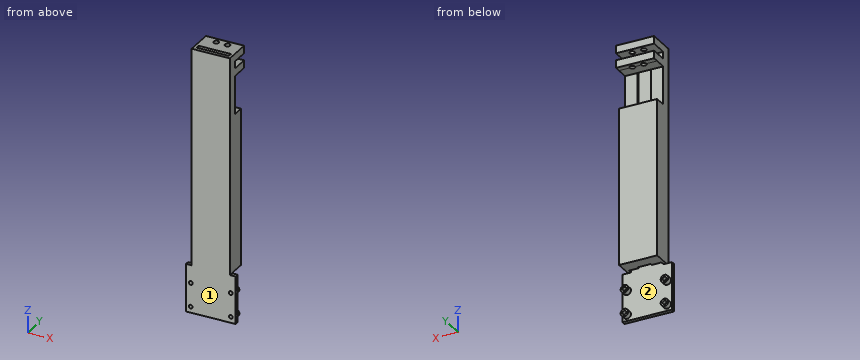
Autodesk Inventor part; units mm, degrees
ref_plane "YZ Plane" through (0, 0, 0) normal (1, 0, 0) x (0, 1, 0)
ref_plane "XZ Plane" through (0, 0, 0) normal (0, 1, 0) x (-1, 0, 0)
ref_plane "XY Plane" through (0, 0, 0) normal (0, 0, 1) x (1, 0, 0)
sketch "スケッチ1" plane through (0, 0, 0) normal (0, 1, 0) x (-1, 0, 0)
  line L0 (8.5, 24.0956) -> (-8.5, 24.0956)
  line L1 (-8.5, 24.0956) -> (-8.5, -85.9044)
  line L2 (-8.5, -85.9044) -> (8.5, -85.9044)
  line L3 (8.5, -85.9044) -> (8.5, 24.0956)
  line L4 (13, -85.9044) -> (-13, -85.9044)
  line L5 (-13, -85.9044) -> (-13, -110.9044)
  line L6 (-13, -110.9044) -> (13, -110.9044)
  line L7 (13, -110.9044) -> (13, -85.9044)
  circle A0 centre (10.5, -95.2644) radius 1
  circle A1 centre (10.5, -107.7644) radius 1
  line L8 (0, -85.9044) -> (0, -110.9044)
  line L9 (-8.5, -85.9044) -> (-8.5, 24.0956)
  circle A2 centre (-10.5, -95.2644) radius 1
  circle A3 centre (-10.5, -107.7644) radius 1
  line L10 (0, -85.9044) -> (0, 24.0956)
  line L11 (10, -85.9044) -> (10, 24.0956)
  line L12 (10, 24.0956) -> (8.5, 24.0956)
  line L13 (-8.5, -85.9044) -> (-8.5, 24.0956)
  line L14 (-10, -85.9044) -> (-10, 24.0956)
  line L15 (-10, 24.0956) -> (-8.5, 24.0956)
  line L16 (10, 24.0956) -> (-10, 24.0956)
  line L17 (8.5, 24.0956) -> (-8.5, 24.0956)
  line L18 (10, 24.0956) -> (-10, 24.0956)
  point P0 (0, 0)
  point P1 (-8.5, 24.0956)
  dimension "d0" = 17
  dimension "d1" = 110
  dimension "d2" = 26
  dimension "d3" = 25
  dimension "d4" = 4.5
  dimension "d5" = 2
  dimension "d6" = 9.36
  dimension "d7" = 2
  dimension "d8" = 12.5
  dimension "d9" = 2.5
  dimension "d10" = 2.5
  dimension "d11" = 13
  dimension "d12" = 1.5
extrude "押し出し1" add sketch "スケッチ1" along normal blind 2 contours L3 L2 L10 L0 | L10 L2 L1 L0 | L4 L7 L6 L8 L2 | L8 L6 L5 L4 L2
extrude "押し出し2" add sketch "スケッチ1" along normal blind 5 contours L12 L11 L4 L3 | L1 L4 L14 L15
sketch "スケッチ2" plane through (-8.5, 2, 24.0956) normal (1, 0, 0) x (0, 0, -1)
  line L0 (0, 0) -> (0, 3)
  line L1 (0, 3) -> (110, 3)
  line L2 (110, 3) -> (110, 2)
  line L3 (110, 2) -> (0, 2)
  line L4 (0, 2) -> (0, 3)
  point P0 (24.0956, -2)
  point P1 (0, 2)
  dimension "d27" = 110
  dimension "d28" = 1
sketch "スケッチ3" plane through (8.5, 2, -85.9044) normal (-1, 0, 0) x (0, 0, 1)
  line L0 (0, 3) -> (110, 3)
  line L1 (0, 3) -> (110, 3)
  line L2 (110, 3) -> (110, 2)
  line L3 (110, 2) -> (0, 2)
  line L4 (0, 2) -> (0, 3)
  point P0 (85.9044, -2)
  dimension "d29" = 110
  dimension "d30" = 1
sketch "スケッチ5" plane through (-10, 0, 24.0956) normal (0, 0, 1) x (1, 0, 0)
  line L0 (0, 0) -> (0, 2)
  line L1 (0, 0) -> (20, 0)
  line L2 (20, 0) -> (20, 14)
  line L3 (20, 14) -> (0, 14)
  line L4 (0, 14) -> (0, 0)
  line L5 (0, 2) -> (1.5, 2)
  line L6 (18.5, 4) -> (13.5, 4)
  line L7 (1.5, 2) -> (18.5, 2)
  line L8 (18.5, 2) -> (18.5, 4)
  line L9 (18.5, 4) -> (1.5, 4)
  line L10 (1.5, 4) -> (1.5, 2)
  circle A0 centre (7, 11) radius 1.375
  circle A1 centre (13, 11) radius 1.375
  point P0 (10, 0)
  point P1 (0, 2)
  dimension "d35" = 20
  dimension "d36" = 14
  dimension "d37" = 2.75
  dimension "d38" = 2.75
  dimension "d39" = 3
  dimension "d40" = 3
  dimension "d41" = 6
  dimension "d42" = 7
extrude "押し出し5" add sketch "スケッチ5" along normal blind 4
extrude "押し出し6" add sketch "スケッチ2" along normal blind 5
extrude "押し出し7" add sketch "スケッチ3" along normal blind 5
sketch "スケッチ6" plane through (-10, 0, 28.0956) normal (0, 0, 1) x (1, 0, 0)
  point P0 (10, 0)
sketch "スケッチ8" plane through (0, 2, 0) normal (0, 1, 0) x (1, 0, 0)
  circle A0 centre (10.5, 107.7644) radius 1
  circle A1 centre (10.5, 107.7644) radius 2
  circle A2 centre (-10.5, 107.7644) radius 1
  circle A3 centre (-10.5, 107.7644) radius 2
  circle A4 centre (-10.5, 95.2644) radius 1
  circle A5 centre (-10.5, 95.2644) radius 2
  line L0 (13, 110.9044) -> (-13, 110.9044)
  line L1 (0, 110.9044) -> (0, 85.9044)
  circle A6 centre (10.5, 95.2644) radius 2
  circle A7 centre (10.5, 95.2644) radius 1
  point P0 (0, 0)
  dimension "d49" = 4
  dimension "d50" = 4
  dimension "d53" = 4
  dimension "d73" = 25
extrude "押し出し8" add sketch "スケッチ8" along normal blind 2.7
extrude "押し出し9" cut sketch "スケッチ1" along normal blind 4.8 contours A2
sketch "スケッチ9" plane through (0, 5, 0) normal (0, 1, 0) x (1, 0, 0)
  line L0 (-10, 85.9044) -> (-10, -24.0956)
  line L1 (10, -24.0956) -> (10, 85.9044)
  line L2 (-10, -20.3956) -> (10, -20.3956)
  line L3 (10, -20.3956) -> (10, -16.3956)
  line L4 (10, -16.3956) -> (-10, -16.3956)
  line L5 (-10, -16.3956) -> (-10, -20.3956)
  line L6 (10, -24.0956) -> (-10, -24.0956)
  point P0 (0, 0)
  point P1 (10, -20.3956)
  dimension "d57" = 3.7
  dimension "d58" = 4
extrude "押し出し10" add sketch "スケッチ9" along normal blind 9 contours L4 L1 L2 L0
sketch "スケッチ10" plane through (3.5, 5, 16.3956) normal (0, 0, -1) x (-1, 0, 0)
  line L0 (0, 0) -> (-6.5, 0)
  line L1 (-6.5, 0) -> (13.5, 0)
  line L2 (13.5, 0) -> (13.5, 6)
  line L3 (13.5, 6) -> (-6.5, 6)
  line L4 (-6.5, 6) -> (-6.5, 0)
  point P0 (3.5, -5)
  dimension "d63" = 20
  dimension "d64" = 6
extrude "押し出し12" add sketch "スケッチ10" along normal blind 102.3
extrude "押し出し13" add sketch "スケッチ10" along normal blind 102
extrude "押し出し11" cut sketch "スケッチ5" against normal blind 8 contours A0 | A1
sketch "スケッチ11" plane through (-4.375, 11, 16.3956) normal (0, 1, 0) x (1, 0, 0)
  line L0 (14.375, -11.7) -> (14.375, 102.3)
  line L1 (14.375, 0.0015) -> (-5.625, 0.0015)
  line L2 (-5.625, 0.0015) -> (-5.625, 20.0015)
  line L3 (-5.625, 20.0015) -> (14.375, 20.0015)
  line L4 (14.375, 20.0015) -> (14.375, 0.0015)
  point P0 (4.375, 16.3956)
  dimension "d69" = 20
  dimension "d70" = 20
extrude "押し出し14" cut sketch "スケッチ11" against normal blind 6
properties part number "MouthCameraBase"
Read the model definition and answer for the solid it produces. Units are mm, in the model's axes. Face numbers are marked on the shaded views. Give positions to 0.01 mm unless a question says otherwise; leave off trailing zeros. Write each loop counter-clockwise with the first axis right and the second up, starting at its lowest first coordinate (ties: lowest second). Pieces come first, ordered by that corner, then holes. Notation, with made-up numbers: M 8.5,-31 L 65.5,-31 A23 cw 65.5,-11 Z; hole C -10.75,-14.75 d10. An arc over 180 degrees is marked long. Put each result on its own line as item: value. Start each with the question number.
1. The part is cut by section B-B, the plane z = -77. Give the vertices of the cut face in (x, y), and give its area (3 significant figures).
2. For a pull along X with two mould halves and no side action, classify the marked faces 1 and 2 as released by +X, released by -X, zero draft, split by the parting line, or undercut.
3. The part is cut by section C-C, the plane z = -1. Give the vertices of the cut face in (x, y), and give its area (3 significant figures).
4. Each of these flat-tipped pins is pushed along its axis until it touches: pin 1 Ø1.9 at (x, z) = (-7, 21.5) entering from +Y; pin 2 Ø4 at (y, z) = (11.5, -71.5) entering from +X; pin 3 Ø10 at (x, z) = (-2.5, -57.5) entering from +Y; pin 4 Ø1.2 at (x, z) = (-10.5, -95.26) entering from -Y. Where does it stop, or does it pass through?
5. The part is cut by section A-A, the plane y = 7.75. Give the vertices of the cut face in (x, z), and give its area (3 significant figures).
6. Consider line 1 along Z through (x, y) = (-4, 8.5); line 2 along Y through (x, z) = (3, 17.2) (3 decimals); line 3 along Z through (x, y) = (-10.5, 3.6). Determine where each line is inside the solid, lowest interval first.
Final values:
1. outline: M -10,0 L 10,0 L 10,11 L -10,11 Z; hole M -8.5,2 L 8.5,2 L 8.5,4 L 3.5,4 L 3.5,5 L -3.5,5 L -3.5,4 L -8.5,4 Z
1. area: 179 mm²
2. face 1: zero draft
2. face 2: undercut
3. outline: M -10,0 L 10,0 L 10,5 L 3.5,5 L 3.5,4 L 8.5,4 L 8.5,2 L -8.5,2 L -8.5,4 L -3.5,4 L -3.5,5 L -10,5 Z
3. area: 59.0 mm²
4. pin 1: stops at y = 5
4. pin 2: stops at x = 10
4. pin 3: stops at y = 11
4. pin 4: passes through
5. outline: M -10,-85.9 L 10,-85.9 L 10,-3.61 L -10,-3.61 Z; M -10,16.39 L 10,16.39 L 10,20.4 L -10,20.4 Z; M -10,24.1 L 10,24.1 L 10,28.1 L -10,28.1 Z
5. area: 1,810 mm²
6. line 1: z = -85.9 to -3.61, 16.39 to 20.4, 24.1 to 28.1
6. line 2: y = 0 to 2, 5 to 9.625, 12.375 to 14
6. line 3: z = -109.76 to -108.76, -106.76 to -105.76, -97.26 to -96.26, -94.26 to -93.26
